Input: part model. Units: mm. Frame: model coordinates. Face numbers are marked on the shaded views. Round coordinates to 2 decimals unless told otherwise and drop trailing zeros. Loops run counter-clockwise (first coordinate to the right, second up) from the corner with the lowest first, then second, coordinate; pieces in that order, holes last. Notation, with made-up numbers: (52, 2.5) -> (89, 2.5) arc R29 cw to (89, 27.5) -> close; hole circle Ø7 at (84.25, 54). An arc over 180 degrees is marked (long way). Answer as a JSON object with one key per item and string values. Group by question number.
Item 1: Material intervals for line 1 (X direction, y = -270.5, z = -17.5); line 2 (Z direction, x = -55.5, y = -271.5); line 3 (X direction, y = -278, z = -57.5), sorted ascending. Write a range as [from, to].
Item 2: Draft query along Z for the marked faces 1, 2, 3 and 4. Return one class per face: released by +Z, released by -Z, zero draft, split by the parting line, or undercut.
Item 3: Section query A-A on z = -69. Return loops of the section in (x, y), and give its area (3 significant figures).
Item 4: Section query D-D on z = -23. Return loops of the section in (x, y), and give its area (3 significant figures).
Item 5: Pin query (flat end, axial travel): pin 1 (0.6 mm diameter, centred on x = 21.5, y = -276, fed in from +Z); pin 2 (1 mm diameter, centred on x = -48.5, y = -266, fed in from +Z); pin 3 (5 mm diameter, centred on y = -265, z = -44, fed in from -X); pin 4 (12 mm diameter, centred on x = -41.5, z = -60, fed in from -Y). Return the tip coordinate at first contact, or that it passes through.
Item 6: Section query C-C on x = -48. Return loops of the section in (y, z), and give its area (3 significant figures).
Item 7: Section query B-B on x = -27. Return loops of the section in (y, z), and give its area (3 significant figures).
from build123d import *

# Parameters (mm, degrees)
TYRE_BASE_SKETCH_R     = 40
TYRE_BASE_DEPTH        = 20
RIM_BORE_SKETCH_R      = 27
RIM_BORE_DEPTH         = 20.2
TREAD_RIB_SKETCH_W     = 3.2
TREAD_RIB_SKETCH_H     = 20
TREAD_RIB_DEPTH        = 4
CIRCULARPATTERN1_COUNT = 12


with BuildPart() as part:
    # Tyre base sketch → Tyre base (new body)
    with BuildSketch(Plane(origin=(0, -283, 0), x_dir=(1, 0, 0), z_dir=(0, 1, 0))):
        with Locations(Location((-19.009182883, 53.244882879, 0), (0, 0, 270))):
            Circle(TYRE_BASE_SKETCH_R)
    extrude(amount=TYRE_BASE_DEPTH)

    # Rim bore sketch → Rim bore (cut)
    with BuildSketch(Plane(origin=(0, -283.1, 0), x_dir=(1, 0, 0), z_dir=(0, 1, 0))):
        with Locations(Location((-19.009182883, 53.244882879, 0), (0, 0, 270))):
            Circle(RIM_BORE_SKETCH_R)
    extrude(amount=RIM_BORE_DEPTH, mode=Mode.SUBTRACT)

    # Tread rib sketch → Tread rib (add)
    with BuildSketch(Plane.XY.offset(-55.244882879)):
        with Locations((20.490817117, -273)):
            Rectangle(TREAD_RIB_SKETCH_W, TREAD_RIB_SKETCH_H)
    tread_rib = extrude(amount=TREAD_RIB_DEPTH)

    # CircularPattern1: Tread rib ×12 about axis
    circularpattern1_axis = Axis((-19.009182883, 0, -53.244882879), (0, 1, 0))
    for i in range(1, CIRCULARPATTERN1_COUNT):
        add(tread_rib.rotate(circularpattern1_axis, i * 360 / CIRCULARPATTERN1_COUNT))


solid = part.part
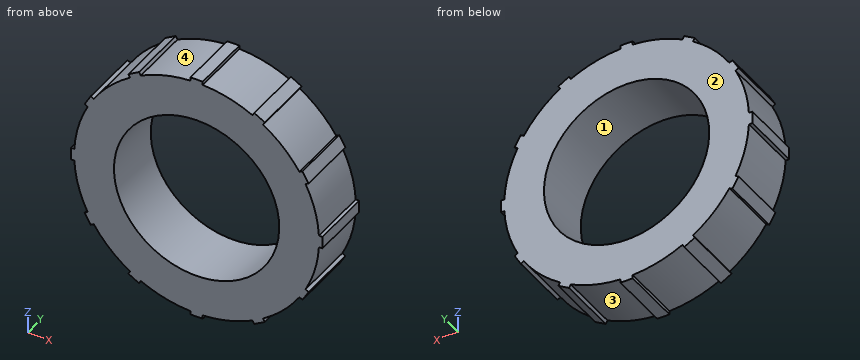
Solved:
{
 "1": {"line 1": "[-39.3, -37.34], [-36.96, -1.06], [-0.68, 1.28]", "line 2": "[-72.24, -72], [-69.63, -36.86], [-34.49, -34.25]", "line 3": "[-58.78, -45.67], [7.65, 20.76]"},
 "2": {"face 1": "undercut", "face 2": "zero draft", "face 3": "released by -Z", "face 4": "released by +Z"},
 "3": {"outline": "(-55.78, -283) -> (-40.94, -283) -> (-40.94, -263) -> (-55.78, -263) -> close; (2.92, -283) -> (17.76, -283) -> (17.76, -263) -> (2.92, -263) -> close", "area": "594 mm²"},
 "4": {"outline": "(-45.19, -283) -> (7.17, -283) -> (7.17, -263) -> (-45.19, -263) -> close", "area": "1,050 mm²"},
 "5": {"pin 1": "z = -51.24", "pin 2": "z = -25.69", "pin 3": "x = -58.44", "pin 4": "y = -283"},
 "6": {"outline": "(-283, -80.8) -> (-263, -80.8) -> (-263, -25.69) -> (-283, -25.69) -> close", "area": "1,100 mm²"},
 "7": {"outline": "(-283, -92.44) -> (-263, -92.44) -> (-263, -79.04) -> (-283, -79.04) -> close; (-283, -27.45) -> (-263, -27.45) -> (-263, -14.05) -> (-283, -14.05) -> close", "area": "536 mm²"}
}
